```python
from build123d import *

# Parameters (mm, degrees)
BOSS_EXTRU_1_DEPTH      = 200
ESQUISSE4_W             = 5
ESQUISSE4_H             = 50
BOSS_EXTRU_4_DEPTH      = 180
BOSS_EXTRU_7_REACH      = 238.046
ESQUISSE5_W             = 10
ESQUISSE5_H             = 10
ENL_V_MAT_EXTRU_1_DEPTH = 10
ESQUISSE6_W             = 20
ESQUISSE6_H             = 10.719834163
ENL_V_MAT_EXTRU_2_DEPTH = 10
SYM_TRIE3_DEPTH         = 10.719834163
SYM_TRIE3_2_DEPTH       = 50
SYM_TRIE3_START         = 10.719834163
SYM_TRIE3_3_DEPTH       = 39.280165837


# Read off the part's stored shape, not the designer's step: Symétrie3
with BuildPart() as part:
    # Esquisse1 → Boss.-Extru.1 (new body)
    with BuildSketch(Plane.XY):
        Polygon((-105.796013405, 0), (84.203986595, 0), (84.203986595, 33.502126335), (-105.796013405, 2), align=None)
    extrude(amount=BOSS_EXTRU_1_DEPTH)

    # Esquisse4 → Boss.-Extru.4 (add)
    with BuildSketch(Plane(origin=(84.203986595, 0, 0), x_dir=(0, 0, -1), z_dir=(1, 0, 0))):
        with Locations((-202.5, 25)):
            Rectangle(ESQUISSE4_W, ESQUISSE4_H)
        with Locations((2.5, 25)):
            Rectangle(ESQUISSE4_W, ESQUISSE4_H)
    extrude(amount=-BOSS_EXTRU_4_DEPTH)

    # Boss.-Extru.7: up to this plane
    boss_extru_7_end = Plane(origin=(-105.796013405, 2, 200), z_dir=(0.16356768062493265, -0.9865321149638162, 0))
    # Esquisse8 → Boss.-Extru.7 (add, up to the surface)
    with BuildSketch(Plane(origin=(0, 50, 0), x_dir=(1, 0, 0), z_dir=(0, 1, 0)), mode=Mode.PRIVATE) as boss_extru_7_sk1:
        Polygon((84.203986595, 0), (-95.796013405, 0), (-95.796013405, -5), align=None)
    boss_extru_7_tool1 = split(extrude(boss_extru_7_sk1.sketch, amount=-BOSS_EXTRU_7_REACH, mode=Mode.PRIVATE), bisect_by=boss_extru_7_end, keep=Keep.BOTH, mode=Mode.PRIVATE)
    add(boss_extru_7_tool1.solids().sort_by_distance((-35.796013, 50, 1.666667))[0])

    # Esquisse5 → Enlèv. mat.-Extru.1 (cut)
    with BuildSketch(Plane(origin=(84.203986595, 0, 0), x_dir=(0, 0, -1), z_dir=(1, 0, 0))):
        with Locations((-200, 5)):
            Rectangle(ESQUISSE5_W, ESQUISSE5_H)
        with Locations((0, 5)):
            Rectangle(ESQUISSE5_W, ESQUISSE5_H)
    extrude(amount=-ENL_V_MAT_EXTRU_1_DEPTH, mode=Mode.SUBTRACT)

    # Esquisse6 → Enlèv. mat.-Extru.2 (cut)
    with BuildSketch(Plane(origin=(0, 0, -5), x_dir=(-1, 0, 0), z_dir=(0, 0, -1))):
        with Locations((95.796013405, 5.359917081)):
            Rectangle(ESQUISSE6_W, ESQUISSE6_H)
    extrude(amount=-ENL_V_MAT_EXTRU_2_DEPTH, mode=Mode.SUBTRACT)

    # Symétrie3 outline → Symétrie3 (cut)
    with BuildSketch(Plane(origin=(0, 0, 0), x_dir=(1, 0, 0), z_dir=(0, 1, 0))):
        Polygon((-95.796013405, -200), (-95.796013405, -205), (-85.796013405, -205), (-85.796013405, -195), (-105.796013405, -195), (-105.796013405, -200), align=None)
    extrude(amount=SYM_TRIE3_DEPTH, mode=Mode.SUBTRACT)

    # Sym_trie3 2 outline → Sym_trie3 2 (add)
    with BuildSketch(Plane(origin=(0, 0, 0), x_dir=(1, 0, 0), z_dir=(0, 1, 0))):
        Polygon((-85.796013405, -195.277777778), (-85.796013405, -200), (84.203986595, -200), align=None)
    extrude(amount=SYM_TRIE3_2_DEPTH)

    # Sym_trie3 3 outline → Sym_trie3 3 (add)
    with BuildSketch(Plane(origin=(0, 0, 0), x_dir=(1, 0, 0), z_dir=(0, 1, 0)).offset(SYM_TRIE3_START)):
        Polygon((-95.796013405, -195), (-95.796013405, -200), (-85.796013405, -200), (-85.796013405, -195.277777778), align=None)
    extrude(amount=SYM_TRIE3_3_DEPTH)


solid = part.part
```
For this review, take the finished solid that the model builds, in its own axes (mm). A direction names the side the tool comes from. Coordinates: 2 decimals unless noted, no trailing zeros. Order: outer loops, then holes, each group sorted by start corner. A loop starts at its lowest first (then second) coordinate and runs counter-clockwise, first axis right, second up. Notation, with made-up numbers: (11, -2.75) -> (35, -2.75) arc R17 cw to (35, 19.25) -> close; hole circle Ø5 at (14.5, -1.5). An arc over 180 degrees is marked (long way). Answer as CSV lines item,"result".
Q1. Clearance check with flat-ended pins moving along their axes: pin 1 Ø4 at (x, z) = (77.5, 198) entering from -Y; pin 2 Ø2.5 at (y, z) = (3, 202) entering from +X; pin 3 Ø5 at (y, z) = (7.5, 202) entering from -X; pin 4 Ø1.6 at (x, y) = (-96, 3) entering from +Z. State where each tip first meets the part, or that it passes through.
Model answer:
pin 1,"stops at y = 0"
pin 2,"stops at x = 74.2"
pin 3,"stops at x = -85.8"
pin 4,"stops at z = 195"
Q2. Wall thickness on line 1 along Z through (x, y) = (-78.5, 12.5); line 2 along Z through (x, y) = (-73.5, 28.5); line 3 along Y through (x, z) = (63, 32.5): over which ranges is each line inside the solid? List them lowest first. Write a range as [from, to].
Model answer:
line 1,"z = [-5, 4.52], [195.48, 205]"
line 2,"z = [-5, 4.38], [195.62, 205]"
line 3,"y = [0, 29.99]"
Q3. We need section A-A (y = 39). State the section outline as (x, z) points.
Model answer:
outline,"(-95.8, -5) -> (84.2, -5) -> (84.2, 0) -> (-95.8, 5) -> close; (-95.8, 195) -> (84.2, 200) -> (84.2, 205) -> (-95.8, 205) -> close"
Q4. We need section C-C (y = 25.5). State the section outline as (x, z) points, plus the area to 3 significant figures.
Model answer:
outline,"(-95.8, -5) -> (84.2, -5) -> (84.2, 205) -> (-95.8, 205) -> (-95.8, 195) -> (35.94, 198.66) -> (35.94, 1.34) -> (-95.8, 5) -> close"
area,"12,300 mm2"
Q5. We need section D-D (z = 43). State the section outline as (x, y) points.
Model answer:
outline,"(-105.8, 0) -> (84.2, 0) -> (84.2, 33.5) -> (-105.8, 2) -> close"
Q6. Draft analysis for pull direction Z (two halves, no side actions). For faces 1 (the face through (-85.796, 5, 0)), 2 (the face through (-93, 2, 5)), 3 (the face through (74.204, 5, 197)), state which applies: released by +Z, released by -Z, zero draft, split by the parting line, or undercut.
Model answer:
face 1,"zero draft"
face 2,"released by -Z"
face 3,"undercut"
Q7. For faces 4 (the face through (79, 5, 195)), 5 (the face through (79, 5, 5)), 6 (the face through (-91, 10.72, 200)), 7 (the face through (78, 5, 200)), 8 (the face through (-7, 50, 201)), list the 3-axis set-ups (+Z, -Z, +X, -X, +Y, -Y) from which the entire face can be reached by the end or side of a thin tool; tool diameter is ignored.
Model answer:
face 4,"+X, -Y"
face 5,"-Z, +X, -Y"
face 6,"+Z, -Z, -X, -Y"
face 7,"+Z, +X, -Y"
face 8,"+Z, -Z, +X, -X, +Y"
Q8. We need section B-B (x = 23.5). State the section outline as (y, z) points.
Model answer:
outline,"(0, -5) -> (50, -5) -> (50, 1.69) -> (23.44, 1.69) -> (23.44, 198.31) -> (50, 198.31) -> (50, 205) -> (0, 205) -> close"
